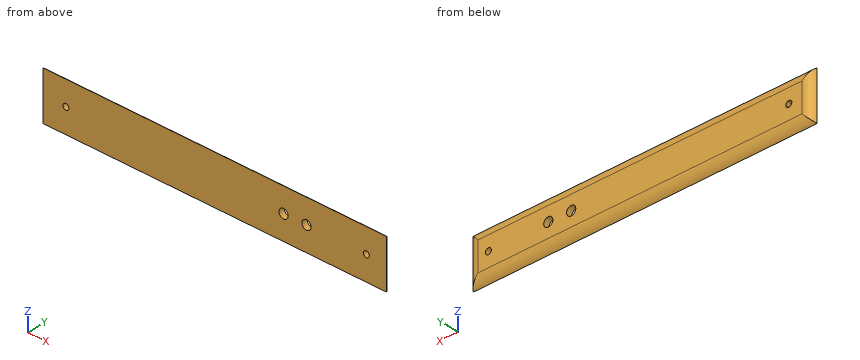
from build123d import *

# Parameters (mm, degrees)
SKETCH_1_W          = 21
SKETCH_1_H          = 42.43
SKETCH_1_R          = 2.6
EXTRUDE_1_DEPTH     = 5
FILLET_1_R          = 10
CUT_EXTRUDE_1_DEPTH = 10


with BuildPart() as part:
    # 草图1 → 凸台-拉伸1 (new body)
    # profile 1 of 3: a face of its own
    with BuildSketch(Plane(origin=(0, 0, 0), x_dir=(1, 0, 0), z_dir=(0, 1, 0))):
        with BuildLine():
            Line((-129, 2.4), (-129, 21.215))
            Line((-129, 21.215), (-150, 21.215))
            Line((-150, 21.215), (-150, -21.215))
            Line((-150, -21.215), (-129, -21.215))
            Line((-129, -21.215), (-129, -2.4))
            ThreePointArc((-129, -2.4), (-132.6, 0), (-129, 2.4))
        make_face()
    # profile 2 of 3: a face of its own
    with BuildSketch(Plane(origin=(0, 0, 0), x_dir=(1, 0, 0), z_dir=(0, 1, 0))):
        with BuildLine():
            Line((129, 21.215), (-129, 21.215))
            Line((-129, 21.215), (-129, 2.4))
            ThreePointArc((-129, 2.4), (-127.836669235, 1.44222051), (-127.4, 0))
            ThreePointArc((-127.4, 0), (-127.836669235, -1.44222051), (-129, -2.4))
            Line((-129, -2.4), (-129, -21.215))
            Line((-129, -21.215), (129, -21.215))
            Line((129, -21.215), (129, 21.215))
        make_face()
    # profile 3 of 3: a face of its own
    with BuildSketch(Plane(origin=(0, 0, 0), x_dir=(1, 0, 0), z_dir=(0, 1, 0))):
        with Locations((139.5, 0)):
            Rectangle(SKETCH_1_W, SKETCH_1_H)
        with Locations(Location((132.3, 0, 0), (0, 0, 270))):
            Circle(SKETCH_1_R, mode=Mode.SUBTRACT)
    extrude(amount=EXTRUDE_1_DEPTH)

    # 圆角1
    # the kernel refuses this fillet: 10 mm, written as the material it takes off along each edge
    with BuildSketch(Plane(origin=(150, 5, 42.865635095), x_dir=(-1, 0, 0), z_dir=(0, 0, -1)), Plane(origin=(-150, 5, -42.865635095), x_dir=(1, 0, 0), z_dir=(0, 0, 1))) as fillet_1_piece_1:
        with BuildLine():
            CenterArc((8.660254038, -10), FILLET_1_R, 90, 60)
            Line((0, -5), (-0.173205081, -4.9))
            ThreePointArc((-0.173205081, -4.9), (-0.2, -2.5), (-0.2, 0))
            Line((-0.2, 0), (0, 0.2))
            Line((0, 0.2), (8.660254038, 0.2))
            Line((8.660254038, 0.2), (8.660254038, 0))
        make_face()
    extrude(amount=85.731270189, mode=Mode.SUBTRACT)
    with BuildSketch(Plane(origin=(-171.650635095, 5, 21.215), x_dir=(0, 0, -1), z_dir=(1, 0, 0))) as fillet_1_piece_2:
        with BuildLine():
            CenterArc((8.660254038, -10), FILLET_1_R, 90, 60)
            Line((0, -5), (-0.173205081, -4.9))
            ThreePointArc((-0.173205081, -4.9), (-0.2, -2.5), (-0.2, 0))
            Line((-0.2, 0), (0, 0.2))
            Line((0, 0.2), (8.660254038, 0.2))
            Line((8.660254038, 0.2), (8.660254038, 0))
        make_face()
    extrude(amount=343.301270189, mode=Mode.SUBTRACT)
    with BuildSketch(Plane(origin=(-171.650635095, 5, -21.215), x_dir=(0, -1, 0), z_dir=(1, 0, 0))) as fillet_1_piece_3:
        with BuildLine():
            CenterArc((10, -8.660254038), FILLET_1_R, 120, 60)
            Line((0, -8.660254038), (-0.2, -8.660254038))
            Line((-0.2, -8.660254038), (-0.2, 0))
            Line((-0.2, 0), (0, 0.2))
            ThreePointArc((0, 0.2), (2.5, 0.2), (4.9, 0.173205081))
            Line((4.9, 0.173205081), (5, 0))
        make_face()
    extrude(amount=343.301270189, mode=Mode.SUBTRACT)

    # 草图2 → 切除-拉伸1 (cut)
    with BuildSketch(Plane(origin=(0, 5, 0), x_dir=(1, 0, 0), z_dir=(0, 1, 0))):
        with BuildLine():
            ThreePointArc((64, 0), (60, 4), (56, 0))
            Line((56, 0), (64, 0))
        make_face()
        with BuildLine():
            Line((64, 0), (56, 0))
            ThreePointArc((56, 0), (60, -4), (64, 0))
        make_face()
        with BuildLine():
            ThreePointArc((84, 0), (80, 4), (76, 0))
            Line((76, 0), (84, 0))
        make_face()
        with BuildLine():
            Line((84, 0), (76, 0))
            ThreePointArc((76, 0), (80, -4), (84, 0))
        make_face()
    extrude(amount=-CUT_EXTRUDE_1_DEPTH, mode=Mode.SUBTRACT)


solid = part.part
Could you check a few things on this model? Use its own coordinates, in mm. Give positions to 0.01 mm unless a question says otherwise; leave off trailing zeros. Order: outer loops, then holes, each group sorted by start corner. A loop starts at its lowest first (then second) coordinate and runs counter-clockwise, first axis right, second up. Notation, with made-up numbers: (64.25, -30.5) -> (111.25, -30.5) arc R18 ccw to (111.25, 0.5) -> close; hole circle Ø10 at (17, 68). An arc over 180 degrees is marked (long way). Answer in a Markdown table with one row per item. Add a question column.
Item 1: Imagine slicing it at B-B (y = 3.65). List the corners of the cut face in (x, z) for me.
Item 2: Please list where these lines run through material, in increasing order: probe 1 along X at (y, z) = (1.15, 1); probe 2 along X at (y, z) = (0.65, -0.5); probe 3 along Z at (x, y) = (-131, 3.9).
Item 3: Imagine slicing it at A-A (x = 80). List the corners of the cut face in (y, z) for me (3 decimals), and give its area (3 significant figures).
Item 4: Imagine slicing it at D-D (z = 9). List the corners of the cut face in (x, y) for me, and give its area (3 significant figures).
Item 5: Imagine slicing it at C-C (x = 132.3). List the corners of the cut face in (y, z) for me (3 decimals), and give its area (3 significant figures).
Item 6: I'm going to push flat-ended pins straight in: P1, Ø3, axis at y = 3, z = -5, coming from the -X side; P2, Ø3, axis at x = 33, y = 3, coming from the -Z side. Where does each tip first touch, or does it pass through?
Result:
| question | item | result |
|---|---|---|
| 1 | outline | (-146.36, -17.57) -> (146.36, -17.57) -> (146.36, 17.57) -> (-146.36, 17.57) -> close; hole circle Ø5.2 at (-130, 0); hole circle Ø8 at (60, 0); hole circle Ø8 at (80, 0); hole circle Ø5.2 at (132.3, 0) |
| 2 | probe 1 | -149.23 to -132.4, -127.6 to 56.13, 63.87 to 76.13, 83.87 to 129.9, 134.7 to 149.23 |
| 2 | probe 2 | -149.59 to -132.55, -127.45 to 56.03, 63.97 to 76.03, 83.97 to 129.75, 134.85 to 149.59 |
| 2 | probe 3 | -17.11 to -2.4, 2.4 to 17.11 |
| 3 | outline | (0, -21.215) arc R10 ccw to (5, -12.555) -> (5, -4) -> (0, -4) -> close; (0, 4) -> (5, 4) -> (5, 12.555) arc R10 ccw to (0, 21.215) -> close |
| 3 | area | 147 mm2 |
| 4 | outline | (-150, 0) -> (150, 0) arc R10 ccw to (141.34, 5) -> (-141.34, 5) arc R10 ccw to start |
| 4 | area | 1,470 mm2 |
| 5 | outline | (0, -21.215) arc R10 ccw to (5, -12.555) -> (5, -2.6) -> (0, -2.6) -> close; (0, 2.6) -> (5, 2.6) -> (5, 12.555) arc R10 ccw to (0, 21.215) -> close |
| 5 | area | 161 mm2 |
| 6 | P1 | x = -148.94 |
| 6 | P2 | z = -20.15 |
